For this review, take the finished solid that the model builds, in its own axes (mm). Coordinates: 2 decimals unless noted, no trailing zeros.
1) Insertion check: P1, Ø4, axis at x = -751, y = 0, coming from the -Z side; P2, Ø6.5, axis at x = -566, y = 0, coming from the -Z side; P3, Ø5, axis at y = -0.5, z = 9, coming from the -X side. Each pin has a flat end and moves straight along its axis. Give the tip position at first contact, or say it passes through.
2) To check wall thickness, follow line 1 along Y through (x, z) = (419, 9); line 2 along Z through (x, y) = (221, -12.4); line 3 along Y through (x, z) = (-243, -5.25). State the ranges of each line that lie inside material, in increasing order.
3) We need section A-A on x = -353.5. Give the number of separate pieces and of enclosed holes in the cut face, then the cut area to 3 significant figures.
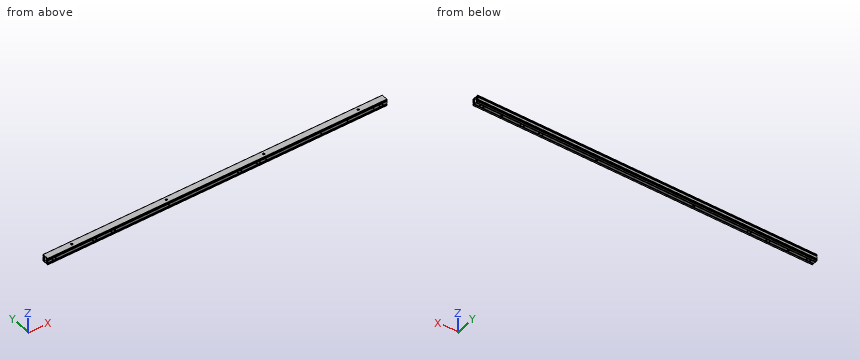
from build123d import *

# Parameters (mm, degrees)
SKETCH_1_W             = 23.5
SKETCH_1_H             = 12
EXTRUDE_1_DEPTH        = 771
HOLE_WIZARD_M6_1_D     = 5
HOLE_WIZARD_M6_1_DEPTH = 15
HOLE_WIZARD_M6_1_TIP   = 1.502151548
HOLE_WIZARD_M6_2_D     = 5
HOLE_WIZARD_M6_2_DEPTH = 15
HOLE_WIZARD_M6_2_TIP   = 1.502151548
SKETCH_6_R             = 4.5
CUT_EXTRUDE_1_DEPTH    = 772.729227126
HOLE_WIZARD_M4_1_D     = 3.3
HOLE_WIZARD_M4_1_DEPTH = 10.1
HOLE_WIZARD_M4_1_TIP   = 0.991420021
HOLE_WIZARD_M6_3_D     = 5
HOLE_WIZARD_M6_3_DEPTH = 15
HOLE_WIZARD_M6_3_TIP   = 1.502151548


with BuildPart() as part:
    # 草图1 → 凸台-拉伸1 (new, symmetric)
    with BuildSketch(Plane(origin=(0, 0, 0), x_dir=(0, 0, -1), z_dir=(1, 0, 0))):
        with BuildLine():
            Line((-14, 15), (-11.5, 15))
            Line((-11.5, 15), (-11.5, 13.5))
            Line((-11.5, 13.5), (-11.4, 13.5))
            ThreePointArc((-11.4, 13.5), (-11.117157288, 13.382842712), (-11, 13.1))
            Line((-11, 13.1), (-11, 12))
            Line((-11, 12), (-9.5, 12))
            Line((-9.5, 12), (-9.5, 15))
            Line((-9.5, 15), (-8, 15))
            Line((-8, 15), (-8, 12.5))
            Line((-8, 12.5), (-5, 12.5))
            Line((-5, 12.5), (-5, 15))
            Line((-5, 15), (5, 15))
            Line((5, 15), (5, 12.5))
            Line((5, 12.5), (8, 12.5))
            Line((8, 12.5), (8, 15))
            Line((8, 15), (9.5, 15))
            Line((9.5, 15), (9.5, 12))
            Line((9.5, 12), (11, 12))
            Line((11, 12), (11, 13.1))
            ThreePointArc((11, 13.1), (11.117157288, 13.382842712), (11.4, 13.5))
            Line((11.4, 13.5), (11.5, 13.5))
            Line((11.5, 13.5), (11.5, 15))
            Line((11.5, 15), (14, 15))
            ThreePointArc((14, 15), (14.707106781, 14.707106781), (15, 14))
            Line((15, 14), (15, 8))
            Line((15, 8), (12.5, 8))
            Line((12.5, 8), (12.5, 5))
            Line((12.5, 5), (15, 5))
            Line((15, 5), (15, -5))
            Line((15, -5), (12.5, -5))
            Line((12.5, -5), (12.5, -8))
            Line((12.5, -8), (15, -8))
            Line((15, -8), (15, -14))
            ThreePointArc((15, -14), (14.707106781, -14.707106781), (14, -15))
            Line((14, -15), (11.5, -15))
            Line((11.5, -15), (11.5, -13.5))
            Line((11.5, -13.5), (11.4, -13.5))
            ThreePointArc((11.4, -13.5), (11.117157288, -13.382842712), (11, -13.1))
            Line((11, -13.1), (11, -12))
            Line((11, -12), (9.5, -12))
            Line((9.5, -12), (9.5, -15))
            Line((9.5, -15), (8, -15))
            Line((8, -15), (8, -12.5))
            Line((8, -12.5), (5, -12.5))
            Line((5, -12.5), (5, -15))
            Line((5, -15), (-5, -15))
            Line((-5, -15), (-5, -12.5))
            Line((-5, -12.5), (-8, -12.5))
            Line((-8, -12.5), (-8, -15))
            Line((-8, -15), (-9.5, -15))
            Line((-9.5, -15), (-9.5, -12))
            Line((-9.5, -12), (-11, -12))
            Line((-11, -12), (-11, -13.1))
            ThreePointArc((-11, -13.1), (-11.117157288, -13.382842712), (-11.4, -13.5))
            Line((-11.4, -13.5), (-11.5, -13.5))
            Line((-11.5, -13.5), (-11.5, -15))
            Line((-11.5, -15), (-14, -15))
            ThreePointArc((-14, -15), (-14.707106781, -14.707106781), (-15, -14))
            Line((-15, -14), (-15, 14))
            ThreePointArc((-15, 14), (-14.707106781, 14.707106781), (-14, 15))
        make_face()
        with BuildLine():
            Line((12, -10.5), (12, -8.5))
            ThreePointArc((12, -8.5), (11.853553391, -8.146446609), (11.5, -8))
            Line((11.5, -8), (-11.5, -8))
            ThreePointArc((-11.5, -8), (-11.853553391, -8.146446609), (-12, -8.5))
            Line((-12, -8.5), (-12, -10.5))
            ThreePointArc((-12, -10.5), (-11.853553391, -10.853553391), (-11.5, -11))
            Line((-11.5, -11), (11.5, -11))
            ThreePointArc((11.5, -11), (11.853553391, -10.853553391), (12, -10.5))
        make_face(mode=Mode.SUBTRACT)
        with BuildLine():
            Line((-11.5, 11), (11.5, 11))
            ThreePointArc((11.5, 11), (11.853553391, 10.853553391), (12, 10.5))
            Line((12, 10.5), (12, 8.5))
            ThreePointArc((12, 8.5), (11.853553391, 8.146446609), (11.5, 8))
            Line((11.5, 8), (-11.5, 8))
            ThreePointArc((-11.5, 8), (-11.853553391, 8.146446609), (-12, 8.5))
            Line((-12, 8.5), (-12, 10.5))
            ThreePointArc((-12, 10.5), (-11.853553391, 10.853553391), (-11.5, 11))
        make_face(mode=Mode.SUBTRACT)
        Rectangle(SKETCH_1_W, SKETCH_1_H, mode=Mode.SUBTRACT)
    extrude(amount=EXTRUDE_1_DEPTH, both=True)

    # M6 螺纹孔1
    with Locations(Plane.XZ.offset(15)):
        with Locations((-751, 0), (-736, 0), (-566, 0), (-551, 0), (-481, 0), (-466, 0), (94, 0), (109, 0), (179, 0), (194, 0), (736, 0), (751, 0)):
            Hole(HOLE_WIZARD_M6_1_D / 2, depth=HOLE_WIZARD_M6_1_DEPTH)
            with Locations((0, 0, -(HOLE_WIZARD_M6_1_DEPTH + HOLE_WIZARD_M6_1_TIP / 2))):  # 118° drill point
                Cone(0, HOLE_WIZARD_M6_1_D / 2, HOLE_WIZARD_M6_1_TIP, mode=Mode.SUBTRACT)

    # M6 螺纹孔2
    with Locations(Plane(origin=(0, 0, -15), x_dir=(-1, 0, 0), z_dir=(0, 0, -1))):
        with Locations((751, 0), (736, 0), (566, 0), (551, 0), (481, 0), (466, 0), (-481, 0), (-466, 0), (-551, 0), (-566, 0), (-751, 0), (-736, 0)):
            Hole(HOLE_WIZARD_M6_2_D / 2, depth=HOLE_WIZARD_M6_2_DEPTH)
            with Locations((0, 0, -(HOLE_WIZARD_M6_2_DEPTH + HOLE_WIZARD_M6_2_TIP / 2))):  # 118° drill point
                Cone(0, HOLE_WIZARD_M6_2_D / 2, HOLE_WIZARD_M6_2_TIP, mode=Mode.SUBTRACT)

    # 草图6 → 切除-拉伸1 (cut, through all)
    with BuildSketch(Plane(origin=(0, 0, -15), x_dir=(-1, 0, 0), z_dir=(0, 0, -1))):
        with Locations((-651, 0)):
            Circle(SKETCH_6_R)
        with Locations((-221, 0)):
            Circle(SKETCH_6_R)
        with Locations((221, 0)):
            Circle(SKETCH_6_R)
        with Locations((651, 0)):
            Circle(SKETCH_6_R)
    extrude(amount=-CUT_EXTRUDE_1_DEPTH, mode=Mode.SUBTRACT)

    # M4 螺纹孔1
    with Locations(Plane.XZ.offset(15)):
        with Locations((711, 0), (591, 0), (471, 0), (221, 0)):
            Hole(HOLE_WIZARD_M4_1_D / 2, depth=HOLE_WIZARD_M4_1_DEPTH)
            with Locations((0, 0, -(HOLE_WIZARD_M4_1_DEPTH + HOLE_WIZARD_M4_1_TIP / 2))):  # 118° drill point
                Cone(0, HOLE_WIZARD_M4_1_D / 2, HOLE_WIZARD_M4_1_TIP, mode=Mode.SUBTRACT)

    # M6 螺纹孔3
    with Locations(Plane.XZ.offset(15)):
        with Locations((-221, 0)):
            Hole(HOLE_WIZARD_M6_3_D / 2, depth=HOLE_WIZARD_M6_3_DEPTH)
            with Locations((0, 0, -(HOLE_WIZARD_M6_3_DEPTH + HOLE_WIZARD_M6_3_TIP / 2))):  # 118° drill point
                Cone(0, HOLE_WIZARD_M6_3_D / 2, HOLE_WIZARD_M6_3_TIP, mode=Mode.SUBTRACT)


solid = part.part
Result:
1. P1: stops at z = 11.75
1. P2: stops at z = -15
1. P3: passes through
2. line 1: y = -15 to -11, -8 to -6, 6 to 8, 11 to 15
2. line 2: z = -15 to -11, -9.5 to -1.65, 1.65 to 9.5, 11 to 15
2. line 3: y = -12.5 to -11, -8 to -6, 6 to 8, 11 to 12.5
3. separate pieces: 1
3. enclosed holes: 3
3. area: 407 mm2
